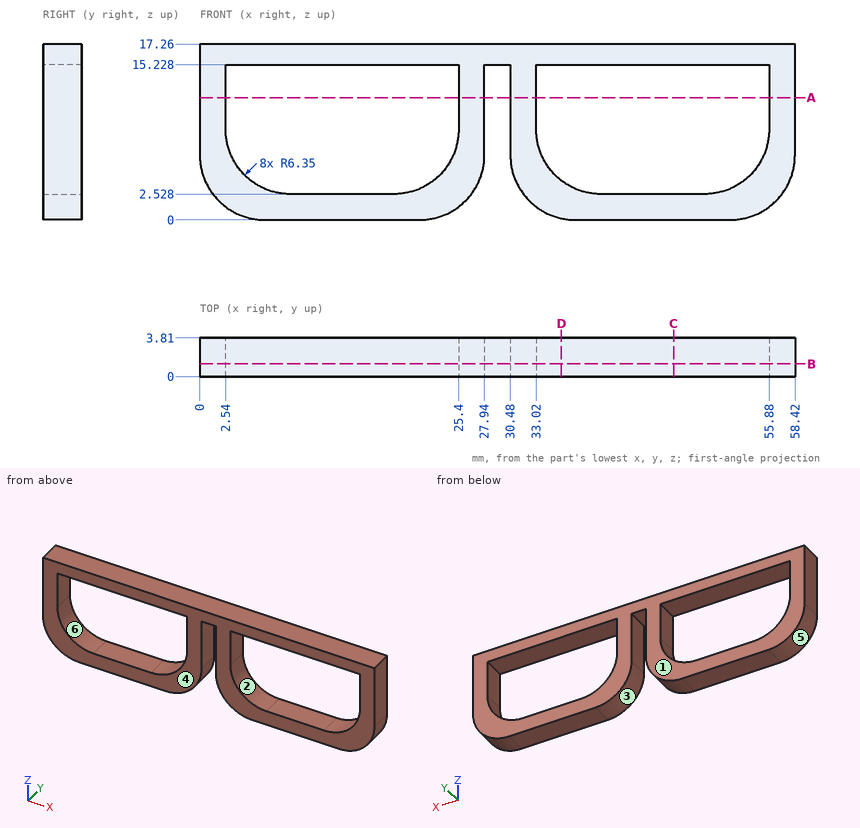
Drawing for the job (mm, zero at the part's lowest x, y, z). A direction names the side the tool comes from. Round coordinates to 2 decimals unless told otherwise and drop trailing zeros. Loops run counter-clockwise (first coordinate to the right, second up) from the corner with the lowest first, then second, coordinate; pieces in that order, holes last. Notation, with made-up numbers: (26, -27.5) - (81, -27.5) arc R26 ccw to (81, 1.5) - close; hole circle Ø6 at (49.5, 21). An arc over 180 degrees is marked (long way). Write each question's results on one line, items separated by ' | '.
(1) Pin check, flat tips, straight feed: pin 1 (1.1 mm diameter, centred on y = 2.5, z = 11, fed in from -X); pin 2 (2 mm diameter, centred on y = 1, z = 4, fed in from -X) (1 decimal); pin 3 (1 mm diameter, centred on x = 33, y = 3, fed in from -Z). Stop position of each tip, or through.
Answer below:
pin 1: stops at x = 0 | pin 2: stops at x = 0.1 | pin 3: stops at z = 0.94
(2) Mould opens along X. For the marked faces 4, 5 and 6 say: released by +X, released by -X, zero draft, split by the parting line, or undercut.
Answer below:
face 4: zero draft | face 5: released by -X | face 6: undercut
(3) Saw through at A-A, the plane z = 12. List the corners of the cut face in (x, y).
Answer below:
outline: (0, 0) - (2.54, 0) - (2.54, 3.81) - (0, 3.81) - close; (25.4, 0) - (27.94, 0) - (27.94, 3.81) - (25.4, 3.81) - close; (30.48, 0) - (33.02, 0) - (33.02, 3.81) - (30.48, 3.81) - close; (55.88, 0) - (58.42, 0) - (58.42, 3.81) - (55.88, 3.81) - close
(4) Wall check: L1, parallel to X at y = 1.15, z = 11.5; L2, parallel to Z at x = 39, y = 2.55; L3, parallel to X at y = 1.25, z = 7.25. Give the ranges that are in metal, low to high.
Answer below:
L1: x = 0 to 2.54, 25.4 to 27.94, 30.48 to 33.02, 55.88 to 58.42 | L2: z = 0 to 2.54, 15.23 to 17.26 | L3: x = 0 to 2.75, 25.19 to 27.94, 30.48 to 33.23, 55.67 to 58.42
(5) Saw through at D-D, the plane x = 35.5. List the corners of the cut face in (y, z).
Answer below:
outline: (0, 0.14) - (3.81, 0.14) - (3.81, 3.84) - (0, 3.84) - close; (0, 15.23) - (3.81, 15.23) - (3.81, 17.26) - (0, 17.26) - close
(6) 3-axis set-ups, long thin cutter, end or side, ignore diameter. For the marked faces 1, 2 and 3: which of +Z, -Z, +X, -X, +Y, -Y reach the whole face in a straight line?
Answer below:
face 1: +Z, -Z, +X, -X, +Y | face 2: +Y, -Y | face 3: -Z, +Y, -Y
(7) Saw through at B-B, the plane y = 1.25. List the corners of the cut face in (x, z), then the cut area to 3 significant figures.
Answer below:
outline: (0, 6.35) arc R6.35 ccw to (6.35, 0) - (21.59, 0) arc R6.35 ccw to (27.94, 6.35) - (27.94, 15.23) - (30.48, 15.23) - (30.48, 6.35) arc R6.35 ccw to (36.83, 0) - (52.07, 0) arc R6.35 ccw to (58.42, 6.35) - (58.42, 17.26) - (0, 17.26) - close; hole (2.54, 8.88) arc R6.35 ccw to (8.89, 2.53) - (19.05, 2.53) arc R6.35 ccw to (25.4, 8.88) - (25.4, 15.23) - (2.54, 15.23) - close; hole (33.02, 8.88) arc R6.35 ccw to (39.37, 2.53) - (49.53, 2.53) arc R6.35 ccw to (55.88, 8.88) - (55.88, 15.23) - (33.02, 15.23) - close | area: 389 mm^2
(8) Saw through at C-C, the plane x = 46.5. List the corners of the cut face in (y, z).
Answer below:
outline: (0, 0) - (3.81, 0) - (3.81, 2.53) - (0, 2.53) - close; (0, 15.23) - (3.81, 15.23) - (3.81, 17.26) - (0, 17.26) - close
